Input: part model. Units: mm. Frame: model coordinates. A direction names the side the tool comes from. Coordinates: 2 decimals unless noted, no trailing zeros. Loops run counter-clockwise (first coordinate to the right, second up) from the corner with the lowest first, then second, coordinate; pieces in that order, holes last. Notation, with made-up numbers: M 23.5,47 L 71.5,47 A23 ccw 71.5,69 Z; hole C -8,71 d3. An arc over 180 degrees is marked long. Use a Markdown table: item, result. Add a question column.
1. Section D-D on x = -60. Output: boundary loops of the cut face in (y, z), then the cut area to 3 significant figures.
2. Section C-C on y = -24.5. Output: boundary loops of the cut face in (x, z).
3. Section A-A on y = 0. Output: boundary loops of the cut face in (x, z).
4. Line query: L1, parallel to Y at x = 0, z = 5.15; L2, parallel to Y at x = -23, z = 0.7; L3, parallel to Y at x = 0, z = 10.25. Output: solid intervals per line, ascending. Write a range as [from, to].
5. Draft query along X for faces 4 (the flat face through (-39.05, -38.93, 3.45)), 5 (the flat face through (-2, -60, 4)), 6 (the flat face through (-21, 1, 7)). Return one class per face: +X half, -X half, draft (parallel to the pull), parting line (faces both ways), or undercut.
6. Pin query (flat end, axial travel): pin 1 (3 mm diameter, centred on y = 16.5, z = 3.5, fed in from -X); pin 2 (1.5 mm diameter, centred on y = 42.5, z = 8, fed in from -X); pin 3 (4 mm diameter, centred on x = -23, y = -10.5, fed in from +Z); pin 4 (1.5 mm diameter, centred on x = -57.5, z = 5, fed in from -Y). Return the tip coordinate at first contact, or that it passes through.
7. Section B-B on x = -37. Output: boundary loops of the cut face in (y, z), then the cut area to 3 significant figures.
8. Set-up query: faces 1 (the flat face through (-5.081, -45.976, 3.919)), 2 (the flat face through (3.48, 60.08, 1.97)), 3 (the cylindrical face through (-27.164, -23.953, 5.077)). Return all of +Z, -Z, +X, -X, +Y, -Y with unobstructed straight access to the full face (end or side cutting, diameter ignored); none if empty.
```python
from build123d import *

# Parameters (mm, degrees)
BOSS_EXTRUDE1_DEPTH            = 7
BOSS_EXTRUDE2_DEPTH            = 5.95
BOSS_EXTRUDE3_DEPTH            = 0.95
CUT_EXTRUDE1_DEPTH             = 105.091810437
CUT_EXTRUDE2_START             = -2.4
SKETCH5_R                      = 3.6
CUT_EXTRUDE2_DEPTH             = 2.4
CBORE_FOR_M5_SHCS1_D           = 6.4
CBORE_FOR_M5_SHCS1_CBORE_D     = 12.8
CBORE_FOR_M5_SHCS1_CBORE_DEPTH = 3
CUT_EXTRUDE3_DEPTH             = 4
F_5_0_5_DIAMETER_HOLE1_D       = 5
CSK_FOR_M4_SFHCS1_AT_2_COUNT   = 2
CSK_FOR_M4_SFHCS1_AT_2_PITCH   = 14
CSK_FOR_M4_SFHCS1_AT_3_COUNT   = 2
CSK_FOR_M4_SFHCS1_AT_3_PITCH   = 19.798989873
CSK_FOR_M4_SFHCS1_AT_4_COUNT   = 2
CSK_FOR_M4_SFHCS1_AT_4_PITCH   = 14


with BuildPart() as part:
    # Sketch1 → Boss-Extrude1 (new body)
    with BuildSketch(Plane.XY):
        with BuildLine():
            Line((-8.626586736, 70.391582661), (-68.626586736, 8.341582661))
            ThreePointArc((-68.626586736, 8.341582661), (-72, 0), (-68.626586736, -8.341582661))
            Line((-68.626586736, -8.341582661), (-8.626586736, -70.391582661))
            ThreePointArc((-8.626586736, -70.391582661), (4.498942052, -73.174725633), (12, -62.05))
            Line((12, -62.05), (12, 62.05))
            ThreePointArc((12, 62.05), (4.498942052, 73.174725633), (-8.626586736, 70.391582661))
        make_face()
    extrude(amount=BOSS_EXTRUDE1_DEPTH)

    # Sketch3 → Boss-Extrude2 (add)
    with BuildSketch(Plane(origin=(0, 0, 7), x_dir=(-1, 0, 0), z_dir=(0, 0, -1))):
        Polygon((-12, 3), (-12, 51), (4.299630176, 51), (10.05, 45.249630176), (10.05, 8.750369824), (4.299630176, 3), align=None)
    extrude(amount=-BOSS_EXTRUDE2_DEPTH)

    # Sketch4 → Boss-Extrude3 (add)
    with BuildSketch(Plane.XY.offset(7)):
        Polygon((12, -51), (12, -3), (-4.299630176, -3), (-10.05, -8.750369824), (-10.05, -45.249630176), (-4.299630176, -51), align=None)
    extrude(amount=BOSS_EXTRUDE3_DEPTH)

    # Sketch2 → Cut-Extrude1 (cut, through all)
    with BuildSketch(Plane(origin=(0, 0, 0), x_dir=(-1, 0, 0), z_dir=(0, 0, -1))):
        Polygon((-34.95, 48), (3.056989489, 48), (7.05, 44.006989489), (7.05, 9.993010511), (3.056989489, 6), (-30.956989489, 6), (-30.956989489, -6), (3.056989489, -6), (7.05, -9.993010511), (7.05, -44.006989489), (3.056989489, -48), (-34.95, -48), align=None)
    extrude(amount=-CUT_EXTRUDE1_DEPTH, mode=Mode.SUBTRACT)

    # Sketch5 → Cut-Extrude2 (cut)
    with BuildSketch(Plane.XY.offset(7).offset(CUT_EXTRUDE2_START)):
        with Locations((-60, 0)):
            Circle(SKETCH5_R)
    extrude(amount=CUT_EXTRUDE2_DEPTH, mode=Mode.SUBTRACT)

    # CBORE for M5 SHCS1 (through all)
    with Locations(Plane(origin=(0, 0, 0), x_dir=(-1, 0, 0), z_dir=(0, 0, -1))):
        with Locations((60, 0)):
            CounterBoreHole(CBORE_FOR_M5_SHCS1_D / 2, CBORE_FOR_M5_SHCS1_CBORE_D / 2, CBORE_FOR_M5_SHCS1_CBORE_DEPTH)

    # Sketch8 → Cut-Extrude3 (cut)
    with BuildSketch(Plane(origin=(0, 0, 0), x_dir=(-1, 0, 0), z_dir=(0, 0, -1))):
        Polygon((-2.309401077, 58.05), (2.309401077, 58.05), (4.618802154, 62.05), (2.309401077, 66.05), (-2.309401077, 66.05), (-4.618802154, 62.05), align=None)
    cut_extrude3 = extrude(amount=-CUT_EXTRUDE3_DEPTH, mode=Mode.SUBTRACT)

    # Ø5.0 (5) Diameter Hole1 (through all)
    with Locations(Plane(origin=(0, 0, 4), x_dir=(-1, 0, 0), z_dir=(0, 0, -1))):
        with Locations((0, 62.05)):
            f_5_0_5_diameter_hole1 = Hole(F_5_0_5_DIAMETER_HOLE1_D / 2)

    # Mirror1: Cut-Extrude3, Ø5.0 (5) Diameter Hole1 across plane
    add(cut_extrude3.mirror(Plane.ZX), mode=Mode.SUBTRACT)
    add(f_5_0_5_diameter_hole1.mirror(Plane.ZX), mode=Mode.SUBTRACT)

    # Sketch12 → CSK for M4 SFHCS1 (revolve, cut)
    with BuildSketch(Plane(origin=(-37, -24.5, 7), x_dir=(0, -1, 0), z_dir=(1, 0, 0))):
        Polygon((0, 0), (0, 7), (2.1, 7), (2.1, 6), (4.2, 3.9), (4.2, 0), align=None)
    csk_for_m4_sfhcs1 = revolve(axis=Axis((-37, -24.5, 13.35), (0, 0, -1)), mode=Mode.SUBTRACT)

    # CSK for M4 SFHCS1 at 2: CSK for M4 SFHCS1 ×2
    with Locations(*[(i * CSK_FOR_M4_SFHCS1_AT_2_PITCH, 0, 0) for i in range(1, CSK_FOR_M4_SFHCS1_AT_2_COUNT)]):
        add(csk_for_m4_sfhcs1, mode=Mode.SUBTRACT)

    # CSK for M4 SFHCS1 at 3: CSK for M4 SFHCS1 ×2
    with Locations(*[Vector(0.7071067811865477, 0.7071067811865474, 0) * (i * CSK_FOR_M4_SFHCS1_AT_3_PITCH) for i in range(1, CSK_FOR_M4_SFHCS1_AT_3_COUNT)]):
        add(csk_for_m4_sfhcs1, mode=Mode.SUBTRACT)

    # CSK for M4 SFHCS1 at 4: CSK for M4 SFHCS1 ×2
    with Locations(*[(0, i * CSK_FOR_M4_SFHCS1_AT_4_PITCH, 0) for i in range(1, CSK_FOR_M4_SFHCS1_AT_4_COUNT)]):
        add(csk_for_m4_sfhcs1, mode=Mode.SUBTRACT)


solid = part.part
```
Answers below:
| question | item | result |
|---|---|---|
| 1 | outline | M -17.26,0 L -6.4,0 L -6.4,3 L -3.2,3 L -3.2,4.6 L -3.6,4.6 L -3.6,7 L -17.26,7 Z; M 3.2,3 L 6.4,3 L 6.4,0 L 17.26,0 L 17.26,7 L 3.6,7 L 3.6,4.6 L 3.2,4.6 Z |
| 1 | area | 176 mm² |
| 2 | outline | M -53,0 L -39.1,0 L -39.1,1 L -41.2,3.1 L -41.2,7 L -53,7 Z; M -34.9,0 L -25.1,0 L -25.1,1 L -27.2,3.1 L -27.2,7 L -32.8,7 L -32.8,3.1 L -34.9,1 Z; M -20.9,0 L -7.05,0 L -7.05,7.95 L -10.05,7.95 L -10.05,7 L -18.8,7 L -18.8,3.1 L -20.9,1 Z |
| 3 | outline | M -72,0 L -66.4,0 L -66.4,3 L -63.2,3 L -63.2,4.6 L -63.6,4.6 L -63.6,7 L -72,7 Z; M -56.8,3 L -53.6,3 L -53.6,0 L 12,0 L 12,7 L -56.4,7 L -56.4,4.6 L -56.8,4.6 Z |
| 4 | L1 | y = [-74.05, -64.55], [-59.55, -48], [-6, 6], [48, 59.55], [64.55, 74.05] |
| 4 | L2 | y = [-55.53, -26.6], [-22.4, -12.6], [-8.4, 55.53] |
| 4 | L3 | y = [3, 6], [48, 51] |
| 5 | face 4 | -X half |
| 5 | face 5 | undercut |
| 5 | face 6 | draft |
| 6 | pin 1 | stops at x = -62.19 |
| 6 | pin 2 | stops at x = -10.05 |
| 6 | pin 3 | passes through |
| 6 | pin 4 | stops at y = -20.62 |
| 7 | outline | M -41.05,0 L -26.6,0 L -26.6,1 L -28.7,3.1 L -28.7,7 L -41.05,7 Z; M -22.4,0 L -12.6,0 L -12.6,1 L -14.7,3.1 L -14.7,7 L -20.3,7 L -20.3,3.1 L -22.4,1 Z; M -8.4,0 L 41.05,0 L 41.05,7 L -6.3,7 L -6.3,3.1 L -8.4,1 Z |
| 7 | area | 474 mm² |
| 8 | face 1 | +Z, -Z, +X |
| 8 | face 2 | -Z |
| 8 | face 3 | +Z |
